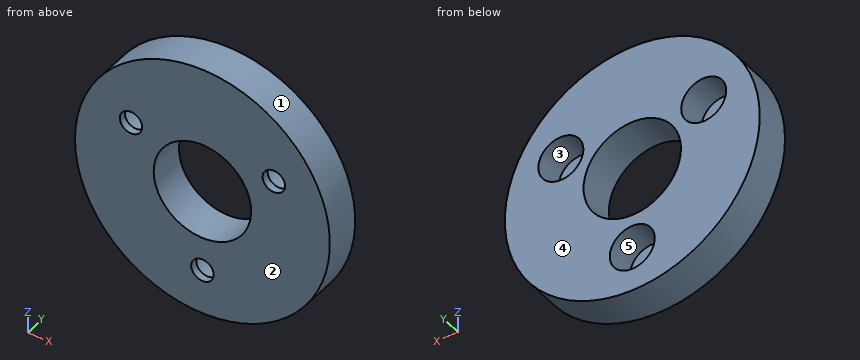
Autodesk Inventor part; units mm, degrees
ref_plane "YZ Plane" through (0, 0, 0) normal (1, 0, 0) x (0, 1, 0)
ref_plane "XZ Plane" through (0, 0, 0) normal (0, 1, 0) x (-1, 0, 0)
ref_plane "XY Plane" through (0, 0, 0) normal (0, 0, 1) x (1, 0, 0)
sketch "Sketch1" plane through (0, 0, 0) normal (0, 0, 1) x (1, 0, 0)
  line L0 (-6.5, 0) -> (-17, 0)
  line L1 (-17, 0) -> (-17, 5)
  line L2 (-17, 5) -> (-6.5, 5)
  line L3 (-6.5, 5) -> (-6.5, 0)
  line L4 (0, -1) -> (0, 6)
  point P0 (0, 0)
  dimension "d0" = 17
  dimension "d1" = 6.5
  dimension "d2" = 5
revolve "Revolution1" add sketch "Sketch1" angle 360 about axis through (0, -10, 0) along (0, 1, 0)
sketch "Sketch3" plane through (0, 5, 0) normal (0, 1, 0) x (1, 0, 0)
  point P0 (0, 0)
  point P1 (0, 11)
  dimension "d16" = 11
hole "Hole2" at (0, 5, -11) direction (0, -1, 0) diameter 3 end through all counterbore diameter 6 counterbore depth 4
pattern_circular "Circular Pattern1" count 3 over 360 about axis through (0, 2.5, 0) along (0, 1, 0) of "Hole2"
properties part number "Insert_Top" material "Brass"
Design review of the part built by this model. Coordinates are the model's own, in mm. Face numbers are marked on the shaded views. A direction names the side the tool comes from. Round coordinates to 2 decimals unless told otherwise and drop trailing zeros. Write each loop counter-clockwise with the first axis right and the second up, starting at its lowest first coordinate (ties: lowest second). Pieces come first, ordered by that corner, then holes. Notation, with made-up numbers: M 64,72 L 74,72 A23 ccw 74,89 Z; hole C 13,40.25 d4. An arc over 180 degrees is marked long. One line per item, written item: value. Start each with the question number.
1. To check wall thickness, follow probe 1 along Z at (x, y) = (0, 4.05); probe 2 along X at (y, z) = (2.1, 5.5); probe 3 along X at (y, z) = (0.4, 5.5). State the ranges of each line that lie inside material, in increasing order. Write a range as from..to.
2. Take a section at D-D on z = 5.5. State the section outline as (x, y) points, then the cut area to 3 significant figures.
3. Take a section at A-A on z = 0. State the section outline as (x, y) points, then the cut area to 3 significant figures.
4. Take a section at B-B on x = 2.5. State the section outline as (y, z) points.
5. Draft analysis for pull direction Z (two halves, no side actions). For the marked faces 1, 2 and 3, state which applies: pulls with the +Z half, pulls with the -Z half, needs draft (parallel to the pull), parting line crosses it, or undercut.
6. Clearance check with flat-ended pins moving along their axes: P1, Ø3, axis at x = 2.5, y = 2, coming from the -Z side; P2, Ø3, axis at y = 3, z = 11, coming from the -X side; P3, Ø1.5, axis at y = 4.5, z = -10, coming from the +X side. State where each tip first meets the part, or that it passes through.
7. Take a section at C-C on y = 3.65. State the section outline as (x, z) points.
8. For the marked faces 4 and 5, list the 3-axis set-ups (+Z, -Z, +X, -X, +Y, -Y) from which the entire face can be reached by the end or side of a thin tool; tool diameter is ignored.
Computed:
1. probe 1: z = -17..-14, -8..-6.5, 6.5..17
1. probe 2: x = -16.09..-12.53, -6.53..-3.46, 3.46..6.53, 12.53..16.09
1. probe 3: x = -16.09..-11.03, -8.03..-3.46, 3.46..8.03, 11.03..16.09
2. outline: M -16.09,0 L -11.03,0 L -11.03,1 L -12.53,1 L -12.53,5 L -16.09,5 Z; M -8.03,0 L -3.46,0 L -3.46,5 L -6.53,5 L -6.53,1 L -8.03,1 Z; M 3.46,0 L 8.03,0 L 8.03,1 L 6.53,1 L 6.53,5 L 3.46,5 Z; M 11.03,0 L 16.09,0 L 16.09,5 L 12.53,5 L 12.53,1 L 11.03,1 Z
2. area: 72.2 mm²
3. outline: M -17,0 L -6.5,0 L -6.5,5 L -17,5 Z; M 6.5,0 L 17,0 L 17,5 L 6.5,5 Z
3. area: 105 mm²
4. outline: M 0,-16.82 L 5,-16.82 L 5,-12.66 L 1,-12.66 L 1,-9.34 L 5,-9.34 L 5,-6 L 0,-6 Z; M 0,6 L 5,6 L 5,16.82 L 0,16.82 Z
5. face 1: parting line crosses it
5. face 2: needs draft
5. face 3: undercut
6. P1: stops at z = -16.97
6. P2: stops at x = -14.1
6. P3: stops at x = 14.26
7. outline: C 0,0 d34; hole C -9.53,5.5 d6; hole C 0,0 d13; hole C 0,-11 d6; hole C 9.53,5.5 d6
8. face 4: +Z, -Z, +X, -X, +Y
8. face 5: +Y
